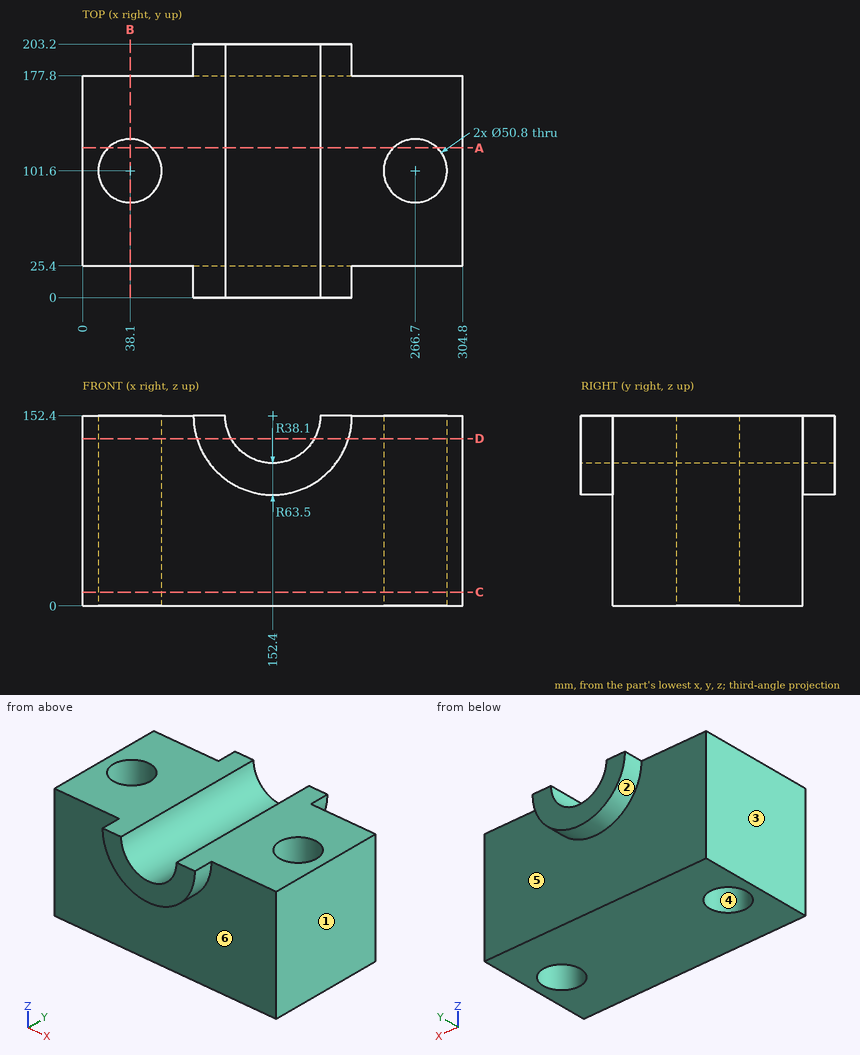
Geometry: see drawing. Coordinates: mm, zero at the bounding-box minimum. A direction names the side the tool comes from. Give positions to 0.01 mm unless a question says otherwise; leave off trailing zeros. Loops run counter-clockwise (first coordinate to the right, second up) from the corner with the lowest first, then second, coordinate; pieces in that order, holes last. Notation, with made-up numbers: (-22.5, -19.75) -> (0.5, -19.75) arc R19 ccw to (0.5, 17.25) -> close; hole circle Ø4 at (41.25, 44). An arc over 180 degrees is marked (long way). Put each result on its own line as item: value.
1. Pin query (flat end, axial travel): P1, Ø4, axis at x = 173, y = 90.5, coming from the +Z side; P2, Ø2, axis at x = 267, z = 60, coming from the -Y side; P3, Ø12, axis at x = 139, z = 80, coming from the +Y side. Return the tip coordinate at first contact, or that it passes through.
Taken from the geometry:
P1: stops at z = 121.73
P2: stops at y = 25.4
P3: stops at y = 177.8
2. Cut plane D-D (z = 134). Return the cut outline in (x, y).
Taken from the geometry:
outline: (0, 25.4) -> (91.62, 25.4) -> (91.62, 0) -> (119.04, 0) -> (119.04, 203.2) -> (91.62, 203.2) -> (91.62, 177.8) -> (0, 177.8) -> close; (185.76, 0) -> (213.18, 0) -> (213.18, 25.4) -> (304.8, 25.4) -> (304.8, 177.8) -> (213.18, 177.8) -> (213.18, 203.2) -> (185.76, 203.2) -> close; hole circle Ø50.8 at (38.1, 101.6); hole circle Ø50.8 at (266.7, 101.6)
3. Ray query, line 1 along X through (y, z) = (101, 45); line 2 along Y through (x, z) = (38.1, 107.5); line 3 along X through (y, z) = (80, 124). Return the intervals inside material, ascending. Write a range as [from, to].
Taken from the geometry:
line 1: x = [0, 12.71], [63.49, 241.31], [292.09, 304.8]
line 2: y = [25.4, 76.2], [127, 177.8]
line 3: x = [0, 24.74], [51.46, 127], [177.8, 253.34], [280.06, 304.8]
4. Pull-direction query (Y, two-part tool) for the marked faces 3, 4, 5 and 6; classes: released by +Y, released by -Y, zero draft, split by the parting line, or undercut.
Taken from the geometry:
face 3: zero draft
face 4: undercut
face 5: released by +Y
face 6: released by -Y
5. Cut plane A-A (y = 120). Return the cut outline in (x, z), plus the area to 3 significant figures.
Taken from the geometry:
outline: (0, 0) -> (20.59, 0) -> (20.59, 152.4) -> (0, 152.4) -> close; (55.61, 0) -> (249.19, 0) -> (249.19, 152.4) -> (190.5, 152.4) arc R38.1 cw to (114.3, 152.4) -> (55.61, 152.4) -> close; (284.21, 0) -> (304.8, 0) -> (304.8, 152.4) -> (284.21, 152.4) -> close
area: 33,500 mm2
6. Set-up query: the marked faces 1 and 2. Return all of +Z, -Z, +X, -X, +Y, -Y with unobstructed straight access to the full face (end or side cutting, diameter ignored); none if empty.
Taken from the geometry:
face 1: +Z, -Z, +X, +Y, -Y
face 2: -Z, +Y
7. Cut plane B-B (x = 38.1). Return the cut outline in (y, z).
Taken from the geometry:
outline: (25.4, 0) -> (76.2, 0) -> (76.2, 152.4) -> (25.4, 152.4) -> close; (127, 0) -> (177.8, 0) -> (177.8, 152.4) -> (127, 152.4) -> close
8. Cut plane C-C (z = 11). Return the cut outline in (x, y), plus the area to 3 significant figures.
Taken from the geometry:
outline: (0, 25.4) -> (304.8, 25.4) -> (304.8, 177.8) -> (0, 177.8) -> close; hole circle Ø50.8 at (38.1, 101.6); hole circle Ø50.8 at (266.7, 101.6)
area: 42,400 mm2
